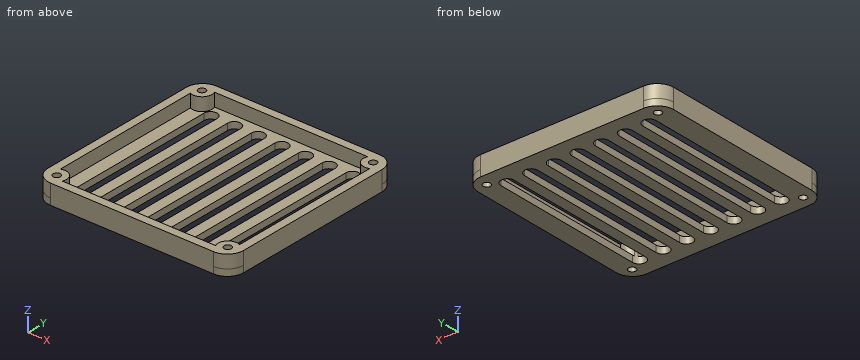
```python
from build123d import *

# Parameters (mm, degrees)
SKETCH1_W           = 120
SKETCH1_H           = 120
SKETCH1_R           = 2.25
BOSS_EXTRUDE1_DEPTH = 4
FILLET1_R           = 10
SKETCH2_R           = 2.25
BOSS_EXTRUDE2_DEPTH = 8
CUT_EXTRUDE1_DEPTH  = 8


with BuildPart() as part:
    # Sketch1 → Boss-Extrude1 (new body)
    with BuildSketch(Plane.XY):
        with Locations((60, 60)):
            Rectangle(SKETCH1_W, SKETCH1_H)
        with Locations((7.5, 112.500076468)):
            Circle(SKETCH1_R, mode=Mode.SUBTRACT)
        with Locations((112.5, 112.500076468)):
            Circle(SKETCH1_R, mode=Mode.SUBTRACT)
        with Locations((7.5, 7.500076468)):
            Circle(SKETCH1_R, mode=Mode.SUBTRACT)
        with Locations((112.373278687, 7.500076468)):
            Circle(SKETCH1_R, mode=Mode.SUBTRACT)
    extrude(amount=BOSS_EXTRUDE1_DEPTH)

    # Fillet1
    fillet1_edges = [part.edges().sort_by_distance(p)[0] for p in [
        (0, 120, 2),
        (120, 120, 2),
        (120, 0, 2),
        (0, 0, 2),
    ]]
    fillet(fillet1_edges, radius=FILLET1_R)

    # Sketch2 → Boss-Extrude2 (add)
    with BuildSketch(Plane.XY.offset(4)):
        with BuildLine():
            Line((0, 110), (0, 10))
            ThreePointArc((0, 10), (2.928932188, 2.928932188), (10, 0))
            Line((10, 0), (110, 0))
            ThreePointArc((110, 0), (117.071067812, 2.928932188), (120, 10))
            Line((120, 10), (120, 110))
            ThreePointArc((120, 110), (117.071067812, 117.071067812), (110, 120))
            Line((110, 120), (10, 120))
            ThreePointArc((10, 120), (2.928932188, 117.071067812), (0, 110))
        make_face()
        with Locations((7.5, 7.500076468)):
            Circle(SKETCH2_R, mode=Mode.SUBTRACT)
        with Locations((112.373278687, 7.500076468)):
            Circle(SKETCH2_R, mode=Mode.SUBTRACT)
        with Locations((112.5, 112.500076468)):
            Circle(SKETCH2_R, mode=Mode.SUBTRACT)
        with Locations((7.5, 112.500076468)):
            Circle(SKETCH2_R, mode=Mode.SUBTRACT)
        with BuildLine():
            Line((5, 107.045720411), (5, 12.954279589))
            ThreePointArc((5, 12.954279589), (11.742610947, 11.742593959), (12.954391106, 5))
            Line((12.954391106, 5), (107.045608894, 5))
            ThreePointArc((107.045608894, 5), (108.257389053, 11.742593959), (115, 12.954279589))
            Line((115, 12.954279589), (115, 107.045720411))
            ThreePointArc((115, 107.045720411), (108.257389053, 108.257406041), (107.045608894, 115))
            Line((107.045608894, 115), (12.954391106, 115))
            ThreePointArc((12.954391106, 115), (11.742610947, 108.257406041), (5, 107.045720411))
        make_face(mode=Mode.SUBTRACT)
    extrude(amount=BOSS_EXTRUDE2_DEPTH)

    # Sketch3 → Cut-Extrude1 (cut)
    with BuildSketch(Plane(origin=(0, 0, 0), x_dir=(-1, 0, 0), z_dir=(0, 0, -1))):
        with BuildLine():
            Line((-100, 107.5), (-100, 12.5))
            ThreePointArc((-100, 12.5), (-104, 8.5), (-108, 12.5))
            Line((-108, 12.5), (-108, 107.5))
            ThreePointArc((-108, 107.5), (-104, 111.5), (-100, 107.5))
        make_face()
        with BuildLine():
            Line((-85.5, 107.5), (-85.5, 12.5))
            ThreePointArc((-85.5, 12.5), (-89.5, 8.5), (-93.5, 12.5))
            Line((-93.5, 12.5), (-93.5, 107.5))
            ThreePointArc((-93.5, 107.5), (-89.5, 111.5), (-85.5, 107.5))
        make_face()
        with BuildLine():
            Line((-71, 107.5), (-71, 12.5))
            ThreePointArc((-71, 12.5), (-75, 8.5), (-79, 12.5))
            Line((-79, 12.5), (-79, 107.5))
            ThreePointArc((-79, 107.5), (-75, 111.5), (-71, 107.5))
        make_face()
        with BuildLine():
            Line((-56.5, 107.5), (-56.5, 12.5))
            ThreePointArc((-56.5, 12.5), (-60.5, 8.5), (-64.5, 12.5))
            Line((-64.5, 12.5), (-64.5, 107.5))
            ThreePointArc((-64.5, 107.5), (-60.5, 111.5), (-56.5, 107.5))
        make_face()
        with BuildLine():
            Line((-42, 107.5), (-42, 12.5))
            ThreePointArc((-42, 12.5), (-46, 8.5), (-50, 12.5))
            Line((-50, 12.5), (-50, 107.5))
            ThreePointArc((-50, 107.5), (-46, 111.5), (-42, 107.5))
        make_face()
        with BuildLine():
            Line((-27.5, 107.5), (-27.5, 12.5))
            ThreePointArc((-27.5, 12.5), (-31.5, 8.5), (-35.5, 12.5))
            Line((-35.5, 12.5), (-35.5, 107.5))
            ThreePointArc((-35.5, 107.5), (-31.5, 111.5), (-27.5, 107.5))
        make_face()
        with BuildLine():
            Line((-13, 107.5), (-13, 12.5))
            ThreePointArc((-13, 12.5), (-17, 8.5), (-21, 12.5))
            Line((-21, 12.5), (-21, 107.5))
            ThreePointArc((-21, 107.5), (-17, 111.5), (-13, 107.5))
        make_face()
    extrude(amount=-CUT_EXTRUDE1_DEPTH, mode=Mode.SUBTRACT)


solid = part.part
```
Part model, mm, in its own coordinate system. Round coordinates to 2 decimals unless told otherwise and drop trailing zeros. Loops run counter-clockwise (first coordinate to the right, second up) from the corner with the lowest first, then second, coordinate; pieces in that order, holes last.
1. Drill centre lines: line 1 along X through (y, z) = (87, 5); line 2 along X through (y, z) = (113, 8.5); line 3 along Y through (x, z) = (112.5, 2.5). Where is each one in solid material? Low to high.
Solutions:
line 1: x = 0 to 5, 115 to 120
line 2: x = 0.46 to 5.31, 9.69 to 13.48, 106.52 to 110.31, 114.69 to 119.54
line 3: y = 0.32 to 5.25, 9.75 to 110.25, 114.75 to 119.68
2. Flat gauge pin, fed straight in: pin 1 (0.7 mm diameter, centred on x = 107, y = 109.5, fed in from -Z). Where does the tip first touch, or does it go through?
Solutions:
pin 1: stops at z = 8
3. Slice it at D-D (x = 7.5). Give the cut face in (y, z).
Solutions:
outline: (0.32, 0) - (5.25, 0) - (5.25, 12) - (0.32, 12) - close; (9.75, 0) - (110.25, 0) - (110.25, 12) - (106.5, 12) - (106.5, 4) - (13.5, 4) - (13.5, 12) - (9.75, 12) - close; (114.75, 0) - (119.68, 0) - (119.68, 12) - (114.75, 12) - close
4. Slice it at B-B (z = 10.25). Give the cut face in (x, y).
Solutions:
outline: (0, 10) arc R10 ccw to (10, 0) - (110, 0) arc R10 ccw to (120, 10) - (120, 110) arc R10 ccw to (110, 120) - (10, 120) arc R10 ccw to (0, 110) - close; hole (5, 12.95) arc R6 cw to (12.95, 5) - (107.05, 5) arc R6 cw to (115, 12.95) - (115, 107.05) arc R6 cw to (107.05, 115) - (12.95, 115) arc R6 cw to (5, 107.05) - close; hole circle Ø4.5 at (7.5, 7.5); hole circle Ø4.5 at (7.5, 112.5); hole circle Ø4.5 at (112.37, 7.5); hole circle Ø4.5 at (112.5, 112.5)
5. Slice it at C-C (y = 78). Count the separate pieces of the cut face and the enclosed holes in it, and give its area (3 significant figures).
Solutions:
separate pieces: 8
enclosed holes: 0
area: 336 mm2
6. Slice it at A-A (x = 60.5). Give the cut face in (y, z).
Solutions:
outline: (0, 0) - (8.5, 0) - (8.5, 4) - (5, 4) - (5, 12) - (0, 12) - close; (111.5, 0) - (120, 0) - (120, 12) - (115, 12) - (115, 4) - (111.5, 4) - close
